from build123d import *

# Parameters (mm, degrees)
EXTRUDE_1_DEPTH                 = 50
SKETCH_2_W                      = 85
SKETCH_2_H                      = 85
CUT_EXTRUDE_1_DEPTH             = 40
SKETCH_3_R                      = 71
CUT_EXTRUDE_2_DEPTH             = 10
EXTRUDE_2_DEPTH                 = 30
PATTERN_CIRCULAR_1_COUNT        = 4
PATTERN_CIRCULAR_1_COPY_1_DEPTH = 30
PATTERN_CIRCULAR_1_COPY_2_DEPTH = 30
SKETCH_8_R                      = 2.5
CUT_EXTRUDE_3_DEPTH             = 30
PATTERN_CIRCULAR_2_COUNT        = 4
CUT_EXTRUDE_4_DEPTH             = 10
SKETCH_10_W                     = 85
SKETCH_10_H                     = 75.258890594
CUT_EXTRUDE_6_DEPTH             = 30
SKETCH_11_W                     = 114
SKETCH_11_H                     = 4.24
EXTRUDE_3_DEPTH                 = 10
SKETCH_12_W                     = 40
SKETCH_12_H                     = 20
CUT_EXTRUDE_7_DEPTH             = 40


with BuildPart() as part:
    # Эскиз1 → Бобышка-Вытянуть1 (new body)
    with BuildSketch(Plane(origin=(0, 0, 0), x_dir=(1, 0, 0), z_dir=(0, 1, 0))):
        with BuildLine():
            Line((-60, -74.613885), (-60, -48.259714048))
            ThreePointArc((-60, -48.259714048), (0, 77), (60, -48.259714048))
            Line((60, -48.259714048), (60, -74.613885))
            Line((60, -74.613885), (60, -122))
            Line((60, -122), (-60, -122))
            Line((-60, -122), (-60, -74.613885))
        make_face()
    extrude(amount=EXTRUDE_1_DEPTH)

    # Эскиз2 → Вырез-Вытянуть1 (cut)
    with BuildSketch(Plane(origin=(0, 50, 0), x_dir=(1, 0, 0), z_dir=(0, 1, 0))):
        Rectangle(SKETCH_2_W, SKETCH_2_H)
    extrude(amount=-CUT_EXTRUDE_1_DEPTH, mode=Mode.SUBTRACT)

    # Эскиз3 → Вырез-Вытянуть2 (cut)
    with BuildSketch(Plane(origin=(0, 50, 0), x_dir=(1, 0, 0), z_dir=(0, 1, 0))):
        Circle(SKETCH_3_R)
    extrude(amount=-CUT_EXTRUDE_2_DEPTH, mode=Mode.SUBTRACT)

    # Эскиз4 → Бобышка-Вытянуть2 (add)
    with BuildSketch(Plane(origin=(0, 50, 0), x_dir=(1, 0, 0), z_dir=(0, 1, 0))):
        with BuildLine():
            Line((0, 71), (0, 77))
            ThreePointArc((0, 77), (-6.710992192, 76.706991753), (-13.37090968, 75.830196982))
            Line((-13.37090968, 75.830196982), (-12.329020614, 69.921350464))
            ThreePointArc((-12.329020614, 69.921350464), (-6.188057735, 70.729823565), (0, 71))
        make_face()
    extrude_2 = extrude(amount=EXTRUDE_2_DEPTH)

    # Зеркальное отражение1: Бобышка-Вытянуть2 across plane
    add(extrude_2.mirror(Plane(origin=(0, 0, 0), x_dir=(0, 0, 1), z_dir=(1, 0, 0))))

    # Круговой массив1: Бобышка-Вытянуть2 ×4 about axis, 1 skipped
    pattern_circular_1_axis = Axis((0, 0, 0), (0, 1, 0))
    add([extrude_2.rotate(pattern_circular_1_axis, i * 360 / PATTERN_CIRCULAR_1_COUNT) for i in range(1, PATTERN_CIRCULAR_1_COUNT) if i not in (2,)])

    # Круговой массив1 copy 1 sketch → Круговой массив1 copy 1 (add)
    with BuildSketch(Plane.ZX.offset(50)):
        with BuildLine():
            Line((0, -71), (0, -77))
            ThreePointArc((0, -77), (-6.710992192, -76.706991753), (-13.37090968, -75.830196982))
            Line((-13.37090968, -75.830196982), (-12.329020614, -69.921350464))
            ThreePointArc((-12.329020614, -69.921350464), (-6.188057735, -70.729823565), (0, -71))
        make_face()
    extrude(amount=PATTERN_CIRCULAR_1_COPY_1_DEPTH)

    # Круговой массив1 copy 2 sketch → Круговой массив1 copy 2 (add)
    with BuildSketch(Plane(origin=(0, 50, 0), x_dir=(0, 0, -1), z_dir=(0, 1, 0))):
        with BuildLine():
            Line((0, -71), (0, -77))
            ThreePointArc((0, -77), (-6.710992192, -76.706991753), (-13.37090968, -75.830196982))
            Line((-13.37090968, -75.830196982), (-12.329020614, -69.921350464))
            ThreePointArc((-12.329020614, -69.921350464), (-6.188057735, -70.729823565), (0, -71))
        make_face()
    extrude(amount=PATTERN_CIRCULAR_1_COPY_2_DEPTH)

    # Эскиз8 → Вырез-Вытянуть3 (cut)
    with BuildSketch(Plane.XY.offset(-70)):
        with Locations((0, 65)):
            Circle(SKETCH_8_R)
    cut_extrude_3 = extrude(amount=-CUT_EXTRUDE_3_DEPTH, mode=Mode.SUBTRACT)

    # Круговой массив2: Вырез-Вытянуть3 ×4 about axis
    pattern_circular_2_axis = Axis((0, 0, 0), (0, 1, 0))
    for i in range(1, PATTERN_CIRCULAR_2_COUNT):
        add(cut_extrude_3.rotate(pattern_circular_2_axis, i * 360 / PATTERN_CIRCULAR_2_COUNT), mode=Mode.SUBTRACT)

    # Эскиз9 → Вырез-Вытянуть4 (cut)
    with BuildSketch(Plane(origin=(0, 50, 0), x_dir=(1, 0, 0), z_dir=(0, 1, 0))):
        Polygon((-57, -68), (-57, -42.5), (57, -42.5), (57, -124), (-57, -124), align=None)
    extrude(amount=-CUT_EXTRUDE_4_DEPTH, mode=Mode.SUBTRACT)

    # Эскиз10 → Вырез-Вытянуть6 (cut)
    with BuildSketch(Plane(origin=(0, 40, 0), x_dir=(1, 0, 0), z_dir=(0, 1, 0))):
        with Locations((0, -80.129445297)):
            Rectangle(SKETCH_10_W, SKETCH_10_H)
    extrude(amount=-CUT_EXTRUDE_6_DEPTH, mode=Mode.SUBTRACT)

    # Эскиз11 → Бобышка-Вытянуть3 (add)
    with BuildSketch(Plane(origin=(0, 40, 0), x_dir=(1, 0, 0), z_dir=(0, 1, 0))):
        with Locations((0, -119.88)):
            Rectangle(SKETCH_11_W, SKETCH_11_H)
    extrude(amount=EXTRUDE_3_DEPTH)

    # Эскиз12 → Вырез-Вытянуть7 (cut)
    with BuildSketch(Plane(origin=(0, 50, 0), x_dir=(1, 0, 0), z_dir=(0, 1, 0))):
        with Locations((-56.627991745, -92)):
            Rectangle(SKETCH_12_W, SKETCH_12_H)
    extrude(amount=-CUT_EXTRUDE_7_DEPTH, mode=Mode.SUBTRACT)


solid = part.part
Here's how the part is built. I have some questions about the finished solid (model axes, mm). A direction names the side the tool comes from. Coordinates: 2 decimals unless noted, no trailing zeros. Loops run counter-clockwise (first coordinate to the right, second up) from the corner with the lowest first, then second, coordinate; pieces in that order, holes last.
1. For P1, Ø1, axis at x = -33, y = 50, coming from the -Z side; P2, Ø4, axis at x = 57.5, y = 46, coming from the -Z side; P3, Ø1, axis at x = -12.5, z = 83, coming from the +Y side; P4, Ø8, axis at x = -28, z = 68, coming from the -Y side, each with a flat end and sliding along its axis, tell me the tip position at first contact or that it passes through.
2. For faces 1 (the flat face through (72.917, 64.79, 12.857)), 2 (the flat face through (12.857, 64.79, -72.917)), 3 (the flat face through (60, 25, 85)), which set-ups out of +Z, -Z, +X, -X, +Y, -Y let a thin tool reach every point of the face, with its end or its side?
3. I need wall thicknesses on L1, parallel to Y at x = 0, z = -73; L2, parallel to X at y = 17.5, z = 74; L3, parallel to X at y = 74.5, z = -1. Which ranges of each line are inside material? Lowest first, please.
4. Imagine slicing it at B-B, the plane y = 65. Please give me the cut outline in (x, z).
5. Imagine slicing it at C-C, the plane x = 49. Please give me the cut outline in (y, z).
6. If we mould it in two halves opening along X, with no side actions, what happens to faces 4 (the flat face through (-60, 25, 77)), 5 (the flat face through (0, 40, -47)), 6 (the flat face through (-51, 26, 102)), 7 (the flat face through (-1, 45, 117.76))? For each: pulls with the +X half, pulls with the -X half, needs draft (parallel to the pull), parting line crosses it, or undercut.
7. Imagine slicing it at A-A, the plane z = 58. Please give me the cut outline in (x, y), and give its area (3 significant figures).
8. Imagine slicing it at D-D, the plane y = 6. Please give me the cut outline in (x, z).
Taken from the geometry:
1. P1: stops at z = -69.81
1. P2: stops at z = -53.37
1. P3: stops at y = 10
1. P4: stops at y = 0
2. face 1: +Z, +Y
2. face 2: +Z, +X, +Y
2. face 3: +Z, +X, +Y, -Y
3. L1: y = 0 to 62.5, 67.5 to 80
3. L2: x = -60 to -42.5, 42.5 to 60
3. L3: x = -76.99 to -70.99, 70.99 to 76.99
4. outline: (-76.96, -2.5) arc R77 ccw to (-75.83, -13.37) - (-69.92, -12.33) arc R71 cw to (-70.96, -2.5) - close; (-76.96, 2.5) - (-70.96, 2.5) arc R71 cw to (-69.92, 12.33) - (-75.83, 13.37) arc R77 ccw to start; (-13.37, -75.83) arc R77 ccw to (-2.5, -76.96) - (-2.5, -70.96) arc R71 cw to (-12.33, -69.92) - close; (2.5, -76.96) arc R77 ccw to (13.37, -75.83) - (12.33, -69.92) arc R71 cw to (2.5, -70.96) - close; (69.92, -12.33) - (75.83, -13.37) arc R77 ccw to (76.96, -2.5) - (70.96, -2.5) arc R71 cw to start; (69.92, 12.33) arc R71 cw to (70.96, 2.5) - (76.96, 2.5) arc R77 ccw to (75.83, 13.37) - close
5. outline: (0, -59.4) - (50, -59.4) - (50, -51.38) - (40, -51.38) - (40, 117.76) - (50, 117.76) - (50, 122) - (0, 122) - close
6. face 4: pulls with the -X half
6. face 5: undercut
6. face 6: needs draft
6. face 7: undercut
7. outline: (-60, 0) - (60, 0) - (60, 50) - (57, 50) - (57, 40) - (42.5, 40) - (42.5, 10) - (-42.5, 10) - (-42.5, 40) - (-57, 40) - (-57, 50) - (-60, 50) - close
7. area: 2,310 mm2
8. outline: (-60, 48.26) arc R77 ccw (long way) to (60, 48.26) - (60, 122) - (-60, 122) - close
